```python
from build123d import *

# Parameters (mm, degrees)
F0_W     = 50.8
F0_H     = 76.2
F2_T     = -2.54
F4_DEPTH = 60.96
F5_R     = 12.7
F6_DEPTH = 49.53


with BuildPart() as f1:
    # F0 (on Front) → F1 (revolve)
    with BuildSketch(Plane.XZ):
        Rectangle(F0_W, F0_H)
    revolve(axis=Axis((-25.4, 0, 0), (0, 0, 1)))

    # F2
    f2_openings = [f1.faces().sort_by_distance(p)[0] for p in [
        (-25.4, 0, -38.1),
    ]]
    offset(amount=F2_T, openings=f2_openings)

    # F3 (on Front) → F4 (cut, symmetric)
    with BuildSketch(Plane.XZ):
        with BuildLine():
            ThreePointArc((8.870553, -38.1), (-25.4, -3.829447), (-59.670553, -38.1))
            Line((-59.670553, -38.1), (8.870553, -38.1))
        make_face()
    extrude(amount=F4_DEPTH, both=True, mode=Mode.SUBTRACT)

    # F5 (on Front) → F6 (join, symmetric)
    with BuildSketch(Plane.XZ):
        with Locations((-25.4, 17.153753)):
            Circle(F5_R)
    extrude(amount=F6_DEPTH, both=True)


solid = f1.part
```
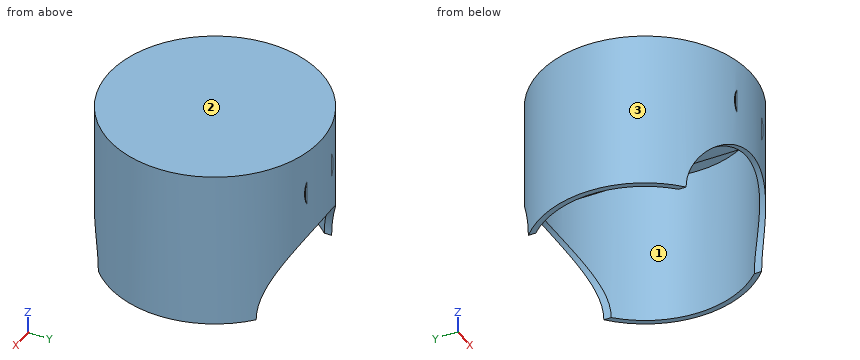
Could you check a few things on this model? Use its own coordinates, in mm. Face numbers are marked on the shaded views. Round coordinates to 2 decimals unless told otherwise and drop trailing zeros. Loops run counter-clockwise (first coordinate to the right, second up) from the corner with the lowest first, then second, coordinate; pieces in that order, holes last. Notation, with made-up numbers: (25.25, -32) - (47.25, -32) arc R17 cw to (47.25, -14) - close; hole circle Ø6 at (2.5, -27). An arc over 180 degrees is marked (long way). Answer in a Markdown table with one row per item. Add a question column.
(1) If we section it at C-C (z = -29.5): Please give me the cut outline in (x, y).
(2) If we section it at A-A (x = -25.4): Please give me the cut outline in (y, z), plus the area to 3 significant figures.
(3) If we section it at B-B (y = -19): Please give me the cut outline in (x, z).
(4) If we section it at D-D (z = -1): Please give me the cut outline in (x, y).
(5) I need wall thicknesses on line 1 along Z through (x, y) = (-60.5, -7.5); line 2 along Y through (x, z) = (-5, 18); line 3 along X through (y, z) = (28, -9). Which ranges of each line are inside material? Lowest first, please.
(6) If we mould it in two halves opening along Y, with no side actions, what happens to the marked faces 1, 2 and 3? For each: pulls with the +Y half, pulls with the -Y half, needs draft (parallel to the pull), parting line crosses it, or undercut.
(7) I'm going to push flat-ended pins straight in: pin 1 (1 mm diameter, centred on x = 13.5, z = -1.5, fed in from +Y); pin 2 (5 mm diameter, centred on x = 6, z = -13, fed in from +Y); pin 3 (0.7 mm diameter, centred on x = -37.5, z = 17.5, fed in from +Y). Where does each tip first touch, or does it pass through?
Model answer:
| question | item | result |
|---|---|---|
| 1 | outline | (-58.57, -38.47) - (-58.57, -35.05) arc R48.26 cw to (-58.57, 35.05) - (-58.57, 38.47) arc R50.8 ccw to start; (7.77, -38.47) arc R50.8 ccw to (7.77, 38.47) - (7.77, 35.05) arc R48.26 cw to (7.77, -35.05) - close |
| 2 | outline | (-50.8, -3.83) - (-48.26, -3.83) - (-48.26, 4.45) - (48.26, 4.45) - (48.26, -3.83) - (50.8, -3.83) - (50.8, 38.1) - (-50.8, 38.1) - close; hole (-48.26, 29.85) - (48.26, 29.85) - (48.26, 35.56) - (-48.26, 35.56) - close |
| 2 | area | 2,910 mm² |
| 3 | outline | (-72.51, -38.1) - (-69.76, -38.1) - (-69.76, 35.56) - (18.96, 35.56) - (18.96, -38.1) - (21.71, -38.1) - (21.71, 38.1) - (-72.51, 38.1) - close; circle Ø25.4 at (-25.4, 17.15) |
| 4 | outline | circle Ø101.6 at (-25.4, 0); hole circle Ø96.52 at (-25.4, 0) |
| 5 | line 1 | z = 35.56 to 38.1 |
| 5 | line 2 | y = -46.52 to -43.74, 43.74 to 46.52 |
| 5 | line 3 | x = -67.79 to -64.71, 13.91 to 16.99 |
| 6 | face 1 | undercut |
| 6 | face 2 | needs draft |
| 6 | face 3 | parting line crosses it |
| 7 | pin 1 | stops at y = 33.26 |
| 7 | pin 2 | stops at y = 41.78 |
| 7 | pin 3 | stops at y = 49.53 |
